Source: three-view drawing plus pictorial views. Frame: mm from the lowest corner of the part. A direction names the side the tool comes from. Round coordinates to 2 decimals unless told otherwise and drop trailing zeros. Loops run counter-clockwise (first coordinate to the right, second up) from the corner with the lowest first, then second, coordinate; pieces in that order, holes last. Notation, with made-up numbers: (24, -0.75) -> (65, -0.75) arc R16 ccw to (65, 7.25) -> close; hole circle Ø7 at (4, -4.5). An arc over 180 degrees is marked (long way). One line per question, with ' | ' between items. Start each with the question number.
Q1. Access query for the marked faces 4 and 5. Directions: +Z, -Z, +X, -X, +Y, -Y. A direction counts if a zero-diameter tool reaches every point of the face in a straight line with its end or side. Return the directions, or none.
Q2. Mould query, pull axis X, two halves, no side actions, for the marked faces 1, 2 and 3. Classes: pulls with the +X half, pulls with the -X half, needs draft (parallel to the pull), parting line crosses it, or undercut.
Q3. Cut plane B-B on z = 268. Return loops of the section in (x, y), and give its area (3 significant figures).
Q4. Material intervals for L1, parallel to X at y = 76.5, z = 268; L2, parallel to X at y = 127, z = 70; L3, parallel to Z at x = 382, y = 21.5, sorted ascending.
Q5. Cut plane C-C on x = 219. Return loops of the section in (y, z).
Q6. Cut plane D-D on x = 293.5. Return loops of the section in (y, z), and give its area (3 significant figures).
Q7. Cut plane A-A on y = 90. State how many separate pieces and enclosed holes the cut face has, and give its area (3 significant figures).
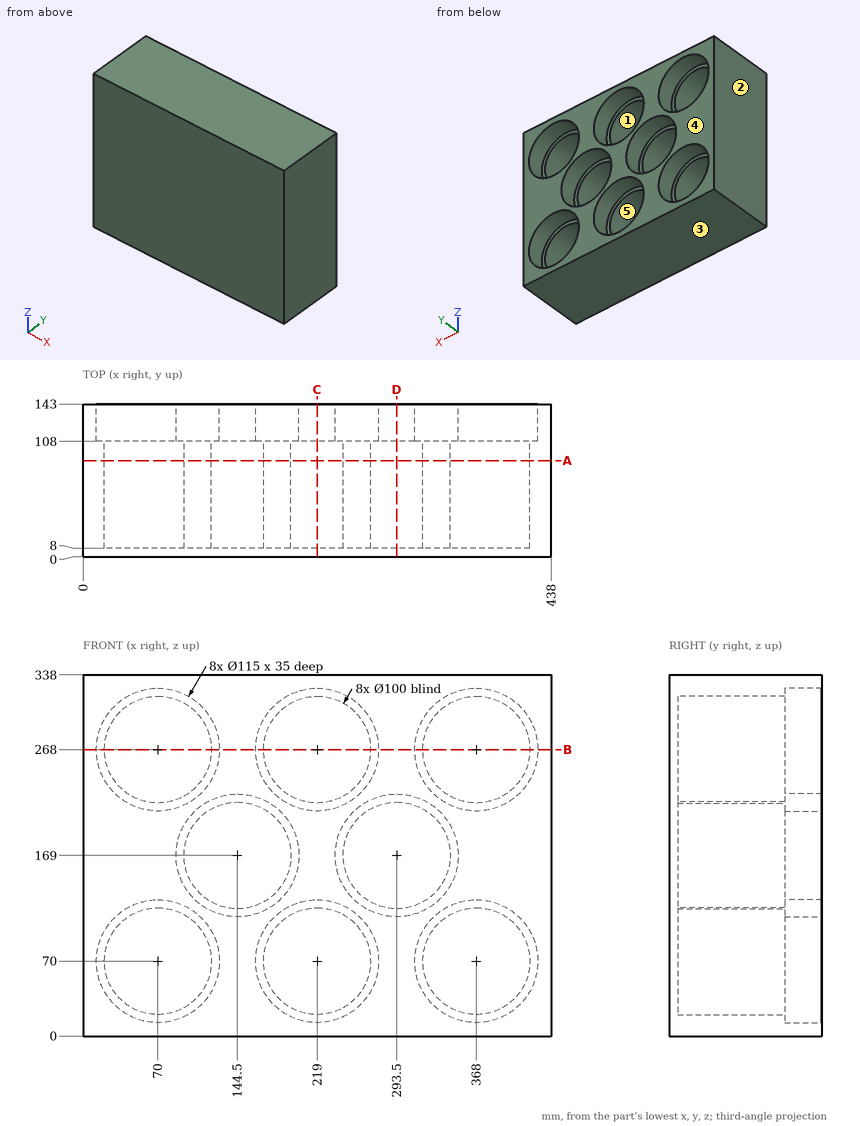
Results:
1) face 4: +Z, -Z, +X, -X, +Y | face 5: +Y
2) face 1: undercut | face 2: pulls with the -X half | face 3: needs draft
3) outline: (0, 0) -> (438, 0) -> (438, 143) -> (425.5, 143) -> (425.5, 108) -> (418, 108) -> (418, 8) -> (318, 8) -> (318, 108) -> (310.5, 108) -> (310.5, 143) -> (276.5, 143) -> (276.5, 108) -> (269, 108) -> (269, 8) -> (169, 8) -> (169, 108) -> (161.5, 108) -> (161.5, 143) -> (127.5, 143) -> (127.5, 108) -> (120, 108) -> (120, 8) -> (20, 8) -> (20, 108) -> (12.5, 108) -> (12.5, 143) -> (0, 143) -> close | area: 20,600 mm^2
4) L1: 0 to 20, 120 to 169, 269 to 318, 418 to 438 | L2: 0 to 12.5, 127.5 to 161.5, 276.5 to 310.5, 425.5 to 438 | L3: 0 to 22, 118 to 220, 316 to 338
5) outline: (0, 0) -> (143, 0) -> (143, 12.5) -> (108, 12.5) -> (108, 20) -> (8, 20) -> (8, 120) -> (108, 120) -> (108, 127.5) -> (143, 127.5) -> (143, 210.5) -> (108, 210.5) -> (108, 218) -> (8, 218) -> (8, 318) -> (108, 318) -> (108, 325.5) -> (143, 325.5) -> (143, 338) -> (0, 338) -> close
6) outline: (0, 0) -> (143, 0) -> (143, 111.5) -> (108, 111.5) -> (108, 119) -> (8, 119) -> (8, 219) -> (108, 219) -> (108, 226.5) -> (143, 226.5) -> (143, 338) -> (0, 338) -> close | area: 34,300 mm^2
7) separate pieces: 1 | enclosed holes: 8 | area: 85,200 mm^2
